Design review of the part built by this model. Coordinates are the model's own, in mm. A direction names the side the tool comes from. Coordinates: 2 decimals unless noted, no trailing zeros. Write each loop counter-clockwise with the first axis right and the second up, starting at its lowest first coordinate (ties: lowest second). Pieces come first, ordered by that corner, then holes.
Q1. The part is to be moulded in two halves that separate along Z. For faces 3 (the cylindrical face through (-0.61, -4.49, 5.48)), 4 (the flat face through (-4.5, 0.1, 0)), 5 (the flat face through (0, 4, 11)), say which applies: released by +Z, released by -Z, zero draft, split by the parting line, or undercut.
Q2. For pin 1 Ø2.5 at (x, z) = (0, 4) entering from -Y, flat-tipped, find the tip position at first contact; note if it passes through.
Q3. For L1, parallel to Y at x = 1.5, z = 14; L2, parallel to X at y = 4.45, z = 4, list the stretches that pass through material, from the lowest coordinate up.
Q4. Take a section at A-A, the plane x = 3.5. Write out the cut boundary in (y, z).
Q5. Take a section at C-C, the plane z = 4. Write out the cut boundary in (x, y), plus the area to 3 significant figures.
Q6. Take a section at D-D, the plane x = 0. Write out the cut boundary in (y, z), plus the area to 3 significant figures.
Q7. For faces 1 (the flat face through (0, -4, 11)), 2 (the flat face through (0, -5, 11)), list the 3-axis set-ups (+Z, -Z, +X, -X, +Y, -Y) from which the entire face can be reached by the end or side of a thin tool; tool diameter is ignored.
from build123d import *

# Parameters (mm, degrees)
SKETCH_281_W          = 10
SKETCH_281_H          = 10
SKETCH_281_W_2        = 8
SKETCH_281_H_2        = 8
EXTRUDE_338_DEPTH     = 23
SKETCH_410_R          = 1.6
CUT_EXTRUDE_739_DEPTH = 26.573423705


with BuildPart() as part:
    # Sketch 281 → Extrude 338 (new body)
    with BuildSketch(Plane.XY):
        Rectangle(SKETCH_281_W, SKETCH_281_H)
        Rectangle(SKETCH_281_W_2, SKETCH_281_H_2, mode=Mode.SUBTRACT)
    extrude(amount=EXTRUDE_338_DEPTH)

    # Sketch 410 → Cut-Extrude 739 (cut, through all)
    with BuildSketch(Plane(origin=(0, 5, 0), x_dir=(1, 0, 0), z_dir=(0, 1, 0))):
        with Locations(Location((0, -4, 0), (0, 0, 270))):
            Circle(SKETCH_410_R)
    extrude(amount=-CUT_EXTRUDE_739_DEPTH, mode=Mode.SUBTRACT)


solid = part.part
Responses:
1. face 3: undercut
1. face 4: released by -Z
1. face 5: zero draft
2. pin 1: passes through
3. L1: y = -5 to -4, 4 to 5
3. L2: x = -5 to -1.6, 1.6 to 5
4. outline: (-5, 0) - (-4, 0) - (-4, 23) - (-5, 23) - close; (4, 0) - (5, 0) - (5, 23) - (4, 23) - close
5. outline: (-5, -5) - (-1.6, -5) - (-1.6, -4) - (-4, -4) - (-4, 4) - (-1.6, 4) - (-1.6, 5) - (-5, 5) - close; (1.6, -5) - (5, -5) - (5, 5) - (1.6, 5) - (1.6, 4) - (4, 4) - (4, -4) - (1.6, -4) - close
5. area: 29.6 mm2
6. outline: (-5, 0) - (-4, 0) - (-4, 2.4) - (-5, 2.4) - close; (-5, 5.6) - (-4, 5.6) - (-4, 23) - (-5, 23) - close; (4, 0) - (5, 0) - (5, 2.4) - (4, 2.4) - close; (4, 5.6) - (5, 5.6) - (5, 23) - (4, 23) - close
6. area: 39.6 mm2
7. face 1: +Z, -Z
7. face 2: +Z, -Z, +X, -X, -Y
